```python
from build123d import *

# Parameters (mm, degrees)
SKETCH_2_R          = 60
SKETCH_2_R_2        = 2.6
SKETCH_2_R_3        = 50
EXTRUDE_1_DEPTH     = 34
CUT_EXTRUDE_START   = -34
SKETCH_3_R          = 2.6
CUT_EXTRUDE_1_DEPTH = 34
FILLET_1_R          = 5


with BuildPart() as part:
    # 草图2 → 凸台-拉伸1 (new body)
    with BuildSketch(Plane.XY):
        Circle(SKETCH_2_R)
        with Locations((0, 55)):
            Circle(SKETCH_2_R_2, mode=Mode.SUBTRACT)
        with Locations((38.890872965, 38.890872965)):
            Circle(SKETCH_2_R_2, mode=Mode.SUBTRACT)
        with Locations((55, 0)):
            Circle(SKETCH_2_R_2, mode=Mode.SUBTRACT)
        with Locations((38.890872965, -38.890872965)):
            Circle(SKETCH_2_R_2, mode=Mode.SUBTRACT)
        with Locations((0, -55)):
            Circle(SKETCH_2_R_2, mode=Mode.SUBTRACT)
        with Locations((-38.890872965, -38.890872965)):
            Circle(SKETCH_2_R_2, mode=Mode.SUBTRACT)
        with Locations((-55, 0)):
            Circle(SKETCH_2_R_2, mode=Mode.SUBTRACT)
        with Locations((-38.890872965, 38.890872965)):
            Circle(SKETCH_2_R_2, mode=Mode.SUBTRACT)
        Circle(SKETCH_2_R_3, mode=Mode.SUBTRACT)
    extrude(amount=EXTRUDE_1_DEPTH)

    # 草图3 → 切除-拉伸1 (cut)
    with BuildSketch(Plane.XY.offset(34).offset(CUT_EXTRUDE_START)):
        with BuildLine():
            Line((55.432771951, 22.961005942), (46.193976626, 19.134171618))
            ThreePointArc((46.193976626, 19.134171618), (49.03926402, 9.754516101), (50, 0))
            ThreePointArc((50, 0), (27.778511651, -41.573480615), (-19.134171618, -46.193976626))
            Line((-19.134171618, -46.193976626), (-22.961005942, -55.432771951))
            ThreePointArc((-22.961005942, -55.432771951), (33.334213981, -49.888176738), (60, 0))
            ThreePointArc((60, 0), (58.847116824, 11.705419321), (55.432771951, 22.961005942))
        make_face()
        with Locations((0, -55)):
            Circle(SKETCH_3_R, mode=Mode.SUBTRACT)
        with Locations((38.890872965, -38.890872965)):
            Circle(SKETCH_3_R, mode=Mode.SUBTRACT)
        with Locations((55, 0)):
            Circle(SKETCH_3_R, mode=Mode.SUBTRACT)
    extrude(amount=CUT_EXTRUDE_1_DEPTH, mode=Mode.SUBTRACT)

    # 圆角1
    fillet_1_edges = [part.edges().sort_by_distance(p)[0] for p in [
        (-19.134171618, -46.193976626, 17),
        (50.813374288, 21.04758878, 34),
        (46.193976626, 19.134171618, 17),
        (55.432771951, 22.961005942, 17),
        (-21.04758878, -50.813374288, 0),
        (-22.961005942, -55.432771951, 17),
        (50.813374288, 21.04758878, 0),
        (-21.04758878, -50.813374288, 34),
    ]]
    fillet(fillet_1_edges, radius=FILLET_1_R - 0.0001)  # a hair under: the kernel refuses the full size


solid = part.part
```
The model under review builds one solid part; all positions refer to its coordinate system, in mm. Give positions to 0.01 mm unless a question says otherwise; leave off trailing zeros. Write each loop counter-clockwise with the first axis right and the second up, starting at its lowest first coordinate (ties: lowest second). Pieces come first, ordered by that corner, then holes.
(1) For P1, Ø2, axis at x = 18.5, z = 25, coming from the +Y side; P2, Ø6, axis at x = -30, z = 27, coming from the +Y side; P3, Ø12, axis at x = -13, z = 7, coming from the -Y side, all flat-tipped, find the tip position at first contact; note any pin that passes through.
(2) Consider section B-B, the plane x = 0. Give the boundary of the cut face in (y, z).
(3) To check wall thickness, follow L1, parallel to Y at x = 0, z = 23; L2, parallel to Y at x = -40, z = 18.5; L3, parallel to X at y = 26.5, z = 5. State the ranges of each line that lie inside material, in increasing order.
(4) Consider section C-C, the plane z = 27. Give the number of separate pieces and of enclosed holes in the cut face, and give its area (3 significant figures).
(5) Consider section A-A, the plane y = 0. Give the boundary of the cut face in (x, z).
(6) Consider section D-D, the plane x = 26.5. Give the boundary of the cut face in (y, z), and give its area (3 significant figures).
(7) The part is to be moulded in two halves that separate along Y. For faces 1 (the flat face through (-41, 33, 0)), 2 (the cylindrical face through (49.7, 22.9, 0.9)), 3 (the cylindrical face through (38.55, 41.47, 16.76)), say which applies: released by +Y, released by -Y, zero draft, split by the parting line, or undercut.
Returned:
1. P1: stops at y = 57.39
1. P2: stops at y = 53.58
1. P3: stops at y = 46.25
2. outline: (50, 0) - (52.4, 0) - (52.4, 34) - (50, 34) - close; (57.6, 0) - (60, 0) - (60, 34) - (57.6, 34) - close
3. L1: y = 50 to 52.4, 57.6 to 60
3. L2: y = -44.72 to -41.24, -36.54 to -30, 30 to 36.54, 41.24 to 44.72
3. L3: x = -53.83 to -42.4, 42.4 to 53.6
4. separate pieces: 1
4. enclosed holes: 5
4. area: 2,030 mm2
5. outline: (-60, 0) - (-57.6, 0) - (-57.6, 34) - (-60, 34) - close; (-52.4, 0) - (-50, 0) - (-50, 34) - (-52.4, 34) - close
6. outline: (42.4, 0) - (53.83, 0) - (53.83, 34) - (42.4, 34) - close
6. area: 389 mm2
7. face 1: zero draft
7. face 2: released by -Y
7. face 3: undercut
